Autodesk Inventor part; units mm, degrees
ref_plane "YZ Plane" through (0, 0, 0) normal (1, 0, 0) x (0, 1, 0)
ref_plane "XZ Plane" through (0, 0, 0) normal (0, 1, 0) x (-1, 0, 0)
ref_plane "XY Plane" through (0, 0, 0) normal (0, 0, 1) x (1, 0, 0)
sketch "Эскиз1" plane through (0, 0, 0) normal (0, 0, 1) x (1, 0, 0)
  line L0 (-15, 0) -> (-15, 3)
  line L1 (-15, 0) -> (0, 0)
  line L2 (0, 2.3791) -> (0, 0.5542) construction
  arc A0 (0, 5.3) -> (-15, 3) centre (0, -44.763) ccw
  line L3 (0, 0) -> (0, 5.3) construction
  line L4 (0, 5.3) -> (0, 0)
  dimension "d0" = 3
  dimension "d1" = 15
  dimension "d6" = 5.3
revolve "Вращение1" add sketch "Эскиз1" angle 360 about axis through (0, 5.3, 0) along (0, -1, 0)
shell "Оболочка1" thickness 0.5 removed faces 1 at (-4.7094, 0, 0) ; own thickness 0.25 on faces at (-14.9514, 2, 1.207)
fillet "Сопряжение1" radius 1 1 edges at (14.75, 2.5543, 0.0003)
sketch "Эскиз2" plane through (0, 0, 0) normal (0, -1, 0) x (1, 0, 0)
  circle A0 centre (9.875, 10.325) radius 1.1
  circle A1 centre (-9.875, 10.325) radius 1.1
  line L0 (9.875, 10.325) -> (-9.875, 10.325) construction
  line L1 (0, 10.325) -> (0, -14.875) construction
  line L2 (0, -14.875) -> (-9.875, 10.325) construction
  line L3 (0, -14.875) -> (9.875, 10.325) construction
  circle A2 centre (0, -14.875) radius 1.1
  circle A3 centre (0, 0) radius 15
  line L4 (0, -15) -> (0, -14.75)
  circle A4 centre (0, 0) radius 14.75
  point P0 (0, -2.275)
  point P1 (0, -2.275)
  point P2 (-9.4386, 11.3347)
  point P3 (-10.9032, 9.934)
  point P4 (10.9032, 9.934)
  point P5 (9.4386, 11.3347)
  point P6 (-10.9708, 10.2294)
  point P7 (-9.7307, 11.4155)
  point P8 (9.7307, 11.4155)
  point P9 (10.9708, 10.2294)
  point P10 (1.0875, -14.7099)
  point P11 (-1.0875, -14.7099)
  point P12 (-1.0967, -14.9599)
  point P13 (1.0967, -14.9599)
  dimension "d11" = 2.2
  dimension "d12" = 19.75
  dimension "d15" = 25.2
extrude "Выдавливание1" cut sketch "Эскиз2" against normal blind 2 contours A0 A3 | A3 A0 A4 | A3 A1 | A1 A4 A3 | A3 L4 A4 A2 | A2 A4 L4 A3
properties part number "зрачок"
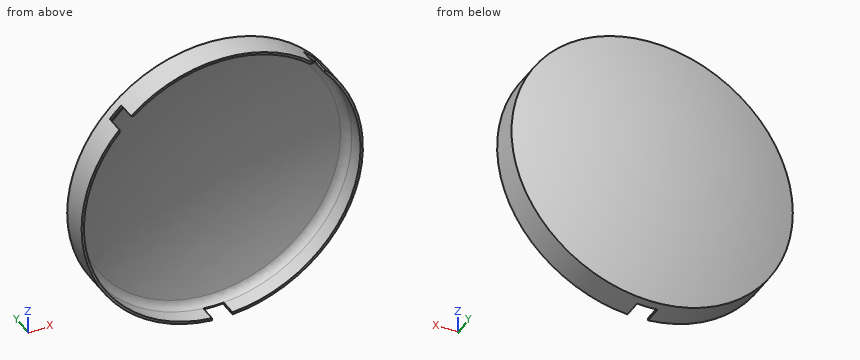
Can you work these out from the model? Positions are in its coordinate system, mm. Coordinates: 2 decimals unless noted, no trailing zeros. Put each result on its own line as item: value. Start each with the question number.
Item 1: For pin 1 (12 mm diameter, centred on x = -2.5, z = 2, fed in from +Y); pin 2 (8 mm diameter, centred on x = 8.5, z = 1.5, fed in from -Y); pin 3 (5 mm diameter, centred on x = -1, z = -8, fed in from +Y); pin 4 (3 mm diameter, centred on y = 3, z = -7.5, fed in from -X), each with a flat end and sliding along its axis, tell me the tip position at first contact or that it passes through.
Item 2: If I drill on line 1 along X through (y, z) = (1.15, -13); line 2 along X through (y, z) = (2.2, -11.75); line 3 along Z through (x, y) = (-5.25, 0.7), over which ranges is the centre line in solid material (lowest first)?
Item 3: Suppose I cut it at A-A (y = 0.5). State how many separate pieces and enclosed holes the cut face has, and give its area (3 significant figures).
Here are the results:
1. pin 1: y = 5.3
1. pin 2: y = 3.16
1. pin 3: y = 4.99
1. pin 4: x = -13.75
2. line 1: -7.48 to -6.97, 6.97 to 7.48
2. line 2: -9.32 to -8.79, 8.79 to 9.32
2. line 3: -14.05 to -13.78, 13.78 to 14.05
3. separate pieces: 3
3. enclosed holes: 0
3. area: 21.9 mm²
